```python
from build123d import *

# Parameters (mm, degrees)
F1_DEPTH = 64.5


with BuildPart() as f1:
    # F0 (on Right) → F1 (new body, symmetric)
    with BuildSketch(Plane.YZ):
        with BuildLine():
            Line((-77, 47), (74, 47))
            ThreePointArc((74, 47), (90.263456, 53.736544), (97, 70))
            Line((97, 70), (97, 284))
            ThreePointArc((97, 284), (90.263456, 300.263456), (74, 307))
            Line((74, 307), (-3, 307))
            Line((-3, 307), (-3, 304))
            Line((-3, 304), (74, 304))
            ThreePointArc((74, 304), (88.142136, 298.142136), (94, 284))
            Line((94, 284), (94, 70))
            ThreePointArc((94, 70), (88.142136, 55.857864), (74, 50))
            Line((74, 50), (-77, 50))
            ThreePointArc((-77, 50), (-93.263456, 43.263456), (-100, 27))
            Line((-100, 27), (-100, 23))
            ThreePointArc((-100, 23), (-93.263456, 6.736544), (-77, 0))
            Line((-77, 0), (97, 0))
            Line((97, 0), (97, 3))
            Line((97, 3), (-77, 3))
            ThreePointArc((-77, 3), (-91.142136, 8.857864), (-97, 23))
            Line((-97, 23), (-97, 27))
            ThreePointArc((-97, 27), (-91.142136, 41.142136), (-77, 47))
        make_face()
    extrude(amount=F1_DEPTH, both=True)


solid = f1.part
```
Design review of the part built by this model. Coordinates are the model's own, in mm. A direction names the side the tool comes from. Round coordinates to 2 decimals unless told otherwise and drop trailing zeros. Write each loop counter-clockwise with the first axis right and the second up, starting at its lowest first coordinate (ties: lowest second). Pieces come first, ordered by that corner, then holes. Notation, with made-up numbers: (79.25, 31) -> (105.25, 31) arc R21 cw to (105.25, 54) -> close; hole circle Ø9 at (86.5, -12). An arc over 180 degrees is marked (long way). Write item = value, one per line. Start each with the question number.
1) Take a section at A-A, the plane y = 12.5. State the section outline as (x, z) points.
2) Take a section at D-D, the plane z = 107. State the section outline as (x, y) points.
3) Clearance check with flat-ended pins moving along their axes: pin 1 (2.5 mm diameter, centred on x = -0.5, z = 305.5, fed in from -Y); pin 2 (4.5 mm diameter, centred on x = -28.5, z = 26, fed in from +Y). State where each tip first meets the part, or that it passes through.
4) Wall thickness on probe 1 along Z at (x, y) = (42, 58); probe 2 along Z at (x, y) = (-2, -26); probe 3 along Z at (x, y) = (0, 88.5): over which ranges is each line inside the solid? List them lowest first. Write a range as from..to.
5) Tool access review of faces 4 (the face through (1, -3, 47)), 5 (the face through (0.903, 87.986, 298.297)), 6 (the face through (1, 36, 307)): name each direction out of +Z, -Z, +X, -X, +Y, -Y from which nothing blocks a thin tool from reaching the whole face with its end or side.
6) Take a section at B-B, the plane y = -11. State the section outline as (x, z) points, plus the area to 3 significant figures.
7) Take a section at C-C, the plane x = 50. State the section outline as (y, z) points, plus the area to 3 significant figures.
8) Mouldability with a two-part tool opening along Z and no side actions: class faces 1 (the face through (0.903, -93.441, 6.916)), 2 (the face through (1, 35, 304)), 3 (the face through (0.903, -93.084, 43.441)) as +Z half, -Z half, draft (parallel to the pull), parting line (faces both ways), or undercut.
Results list:
q1.outline = (-64.5, 0) -> (64.5, 0) -> (64.5, 3) -> (-64.5, 3) -> close; (-64.5, 47) -> (64.5, 47) -> (64.5, 50) -> (-64.5, 50) -> close; (-64.5, 304) -> (64.5, 304) -> (64.5, 307) -> (-64.5, 307) -> close
q2.outline = (-64.5, 94) -> (64.5, 94) -> (64.5, 97) -> (-64.5, 97) -> close
q3.pin_1 = -3
q3.pin_2 = -96.96
q4.probe_1 = 0..3, 47..50, 304..307
q4.probe_2 = 0..3, 47..50
q4.probe_3 = 0..3, 52.15..56.23, 297.77..301.85
q5.face_4 = +X, -X, +Y
q5.face_5 = +X, -X, -Y
q5.face_6 = +Z, +X, -X, +Y, -Y
q6.outline = (-64.5, 0) -> (64.5, 0) -> (64.5, 3) -> (-64.5, 3) -> close; (-64.5, 47) -> (64.5, 47) -> (64.5, 50) -> (-64.5, 50) -> close
q6.area = 774 mm²
q7.outline = (-100, 23) arc R23 ccw to (-77, 0) -> (97, 0) -> (97, 3) -> (-77, 3) arc R20 cw to (-97, 23) -> (-97, 27) arc R20 cw to (-77, 47) -> (74, 47) arc R23 ccw to (97, 70) -> (97, 284) arc R23 ccw to (74, 307) -> (-3, 307) -> (-3, 304) -> (74, 304) arc R20 cw to (94, 284) -> (94, 70) arc R20 cw to (74, 50) -> (-77, 50) arc R23 ccw to (-100, 27) -> close
q7.area = 2,270 mm²
q8.face_1 = -Z half
q8.face_2 = undercut
q8.face_3 = +Z half
